```python
from build123d import *

# Parameters (mm, degrees)
F0_R           = 25
F1_DEPTH       = 25
F3_D           = 2.5
F3_CBORE_D     = 4.5
F3_CBORE_DEPTH = 18


# Not quite as in the source:
# - a fillet or chamfer that OpenCascade refuses, or shapes differently, is made with other operations: its cross-section is extruded or revolved along the edge and cut away or added


with BuildPart() as f1:
    # F0 (on Top) → F1 (new body)
    with BuildSketch(Plane.XY):
        Circle(F0_R)
    extrude(amount=F1_DEPTH)

    # F3 (through all)
    with Locations(Plane.XY.offset(25)):
        with Locations((14.4662138687, 16.5749406124), (14.4662138687, -16.5749406124), (-14.4662138687, -16.5749406124), (-14.4662138687, 16.5749406124)):
            CounterBoreHole(F3_D / 2, F3_CBORE_D / 2, F3_CBORE_DEPTH)

    # F4: fillet of radius 25 on 1 edges, made by hand

    # F4_s1 → F4_t2 (revolve, cut)
    with BuildSketch(Plane.XZ):
        with BuildLine():
            ThreePointArc((25, 0), (17.6776695297, 17.6776695297), (0, 25))
            Line((0, 25), (25, 25))
            Line((25, 25), (25, 0))
        make_face()
    revolve(axis=Axis((0, 0, 25), (0, 0, 1)), mode=Mode.SUBTRACT)


solid = f1.part
```
Can you work these out from the model? Positions are in its coordinate system, mm. A direction names the side the tool comes from. Give positions to 0.01 mm unless a question says otherwise; leave off trailing zeros. Write each loop counter-clockwise with the first axis right and the second up, starting at its lowest first coordinate (ties: lowest second). Pieces come first, ordered by that corner, then holes. Notation, with made-up numbers: (-16, -19.75) -> (33, -19.75) arc R24 ccw to (33, 13.25) -> close; hole circle Ø9 at (42.25, 55). An arc over 180 degrees is marked (long way). One line per item, written item: value.
Q1. Please list where these lines run through material, in increasing order: line 1 (Y direction, x = 15.5, z = 1); line 2 (X direction, y = -15, z = 11.5); line 3 (Y direction, x = -14.5, z = 10). Write a range as [from, to].
Results found:
line 1: y = [-19.59, -17.28], [-15.87, 15.87], [17.28, 19.59]
line 2: x = [-16.36, -16.07], [-12.86, 12.86], [16.07, 16.36]
line 3: y = [-14.33, 14.33]
Q2. Imagine slicing it at B-B on y = 1. Please give me the cut outline in (x, z), and give its area (3 significant figures).
Results found:
outline: (-24.98, 0) -> (24.98, 0) arc R24.98 ccw to start
area: 980 mm^2
Q3. Imagine slicing it at D-D on z = 2.25. Please give me the cut outline in (x, y).
Results found:
outline: circle Ø49.8 at (0, 0); hole circle Ø2.5 at (-14.47, -16.57); hole circle Ø2.5 at (-14.47, 16.57); hole circle Ø2.5 at (14.47, -16.57); hole circle Ø2.5 at (14.47, 16.57)
Q4. Which directions (+Z, -Z, +X, -X, +Y, -Y) give clear straight access to the entire face, cutting with the end or side of a thin tool? Please do faces 4 (the face through (13.31, -17.05, 3.45)), 5 (the face through (-13, 16, 7)).
Results found:
face 4: +Z, -Z
face 5: +Z
Q5. For P1, Ø3, axis at x = 14.47, y = -16.57, coming from the +Z side; P2, Ø5, axis at x = 15.5, z = 6.5, coming from the -Y side; P3, Ø8, axis at x = -16.5, y = -16.5, coming from the +Z side; P4, Ø2, axis at x = -14.47, y = -16.57, coming from the +Z side, each with a flat end and sliding along its axis, tell me the tip position at first contact or that it passes through.
Results found:
P1: stops at z = 7
P2: stops at y = -20.5
P3: stops at z = 15.85
P4: passes through
Q6. We'd pull the mould along Y, two halves only. Please class faces 1 (the face through (13, -16, 7)), 2 (the face through (13.05, -14.826, 10.298)), 3 (the face through (0, 0, 0)): +Y half, -Y half, draft (parallel to the pull), parting line (faces both ways), or undercut.
Results found:
face 1: undercut
face 2: undercut
face 3: draft
Q7. Imagine slicing it at C-C on x = -20. Please give me the cut outline in (y, z), and give its area (3 significant figures).
Results found:
outline: (-15, 0) -> (15, 0) arc R15 ccw to start
area: 353 mm^2
Q8. Imagine slicing it at A-A on z = 13.25. Please give me the cut outline in (x, y), and give its area (3 significant figures).
Results found:
outline: (-15.43, -14.54) arc R2.25 cw to (-12.32, -17.25) arc R21.2 ccw to (12.32, -17.25) arc R2.25 cw to (15.43, -14.54) arc R21.2 ccw to (15.43, 14.54) arc R2.25 cw to (12.32, 17.25) arc R21.2 ccw to (-12.32, 17.25) arc R2.25 cw to (-15.43, 14.54) arc R21.2 ccw to start
area: 1,390 mm^2
